Input: part model. Units: mm. Frame: model coordinates. A direction names the side the tool comes from. Round coordinates to 2 decimals unless told otherwise and drop trailing zeros. Loops run counter-clockwise (first coordinate to the right, second up) from the corner with the lowest first, then second, coordinate; pieces in that order, holes last.
1) Draft query along Z for faces 6 (the face through (10.1, -20.7, 5.1)), 7 (the face through (-12.584, -23.813, 5.664)), 8 (the face through (12.584, -23.813, 5.664)), 9 (the face through (12.53, -24.14, 8.1)). Return one class per face: pulls with the +Z half, pulls with the -Z half, needs draft (parallel to the pull), parting line crosses it, or undercut.
2) Access query for faces 1 (the face through (-14.699, 0.843, 0.285)), 2 (the face through (12.53, -19.9, 8.14)), 3 (the face through (14.715, -19.301, 5.014)), 4 (the face through (-10.401, -24.715, 5.014)), 5 (the face through (10.401, -19.285, 4.986)). Directions: +Z, -Z, +X, -X, +Y, -Y. A direction counts if a zero-diameter tool reaches every point of the face in a straight line with its end or side. Return the directions, or none.
3) Section C-C, the plane z = 6.5. State how many separate pieces and enclosed holes the cut face has, and give its area (3 significant figures).
4) First-contact query: pin 1 (3 mm diameter, centred on x = 3.5, y = 6.5, fed in from +Z); pin 2 (1 mm diameter, centred on x = 13, z = 4.5, fed in from +Y); pin 3 (3 mm diameter, centred on x = 4, z = 6, fed in from +Y). Flat tips, straight axial feed; report the tip coordinate or a pass-through.
5) Section B-B, the plane x = 7.5. Return loops of the section in (y, z).
6) Ray query, line 1 along Y through (x, z) = (-12.75, 6); line 2 along Y through (x, z) = (12.5, 4.25); line 3 along Z through (x, y) = (-12.25, 7). Return the intervals inside material, ascending.
from build123d import *

# Parameters (mm, degrees)
SKETCH1_W           = 30
SKETCH1_H           = 50
BOSS_EXTRUDE1_DEPTH = 3
SKETCH2_W           = 4.9
SKETCH2_H           = 6
BOSS_EXTRUDE2_DEPTH = 6
SKETCH3_R           = 1.55
CUT_EXTRUDE1_DEPTH  = 41.074929819
FILLET1_R           = 3
FILLET2_R           = 1


with BuildPart() as part:
    # Sketch1 → Boss-Extrude1 (new body)
    with BuildSketch(Plane.XY):
        Rectangle(SKETCH1_W, SKETCH1_H)
    extrude(amount=BOSS_EXTRUDE1_DEPTH)

    # Sketch2 → Boss-Extrude2 (add)
    with BuildSketch(Plane.XY.offset(3)):
        with Locations((-12.55, -22)):
            Rectangle(SKETCH2_W, SKETCH2_H)
    boss_extrude2 = extrude(amount=BOSS_EXTRUDE2_DEPTH)

    # Sketch3 → Cut-Extrude1 (cut, through all)
    with BuildSketch(Plane.ZY.offset(15)):
        with Locations((6, -22.3)):
            Circle(SKETCH3_R)
    cut_extrude1 = extrude(amount=-CUT_EXTRUDE1_DEPTH, mode=Mode.SUBTRACT)

    # Mirror1: Boss-Extrude2, Cut-Extrude1 across plane
    add(boss_extrude2.mirror(Plane(origin=(0, 0, 0), x_dir=(0, 0, 1), z_dir=(1, 0, 0))))
    add(cut_extrude1.mirror(Plane(origin=(0, 0, 0), x_dir=(0, 0, 1), z_dir=(1, 0, 0))), mode=Mode.SUBTRACT)

    # Fillet1
    fillet1_edges = [part.edges().sort_by_distance(p)[0] for p in [
        (12.55, -19, 9),
        (12.55, -25, 9),
        (-12.55, -19, 9),
        (-12.55, -25, 9),
    ]]
    fillet(fillet1_edges, radius=FILLET1_R - 0.0001)  # a hair under: the kernel refuses the full size

    # Fillet2
    fillet2_edges = [part.edges().sort_by_distance(p)[0] for p in [
        (-15, 3, 3),
        (0, -25, 3),
        (-10.1, -22, 3),
        (-12.55, -19, 3),
        (15, 3, 3),
        (10.1, -22, 3),
        (12.55, -19, 3),
        (0, -25, 0),
        (15, -25, 3.00005),
        (10.1, -25, 4.50005),
        (-10.1, -25, 4.50005),
        (-15, -25, 3.00005),
        (10.1, -19, 4.50005),
        (-15, 0, 0),
        (10.1, -19.878650367, 8.121349633),
        (10.1, -24.121349633, 8.121349633),
        (15, -19, 4.50005),
        (15, -19.878650367, 8.121349633),
        (15, -24.121349633, 8.121349633),
        (-15, -19, 4.50005),
        (-15, -24.121349633, 8.121349633),
        (0, 25, 0),
        (-15, -19.878650367, 8.121349633),
        (-10.1, -19, 4.50005),
        (-10.1, -24.121349633, 8.121349633),
        (-10.1, -19.878650367, 8.121349633),
        (15, 0, 0),
        (0, 25, 3),
    ]]
    fillet(fillet2_edges, radius=FILLET2_R)


solid = part.part
Final values:
1. face 6: needs draft
1. face 7: undercut
1. face 8: undercut
1. face 9: pulls with the +Z half
2. face 1: -Z, -X, +Y, -Y
2. face 2: +Z, +X, -X, +Y
2. face 3: +Z, +X, +Y
2. face 4: +Z, -Y
2. face 5: +Z, +Y
3. separate pieces: 4
3. enclosed holes: 0
3. area: 27.5 mm2
4. pin 1: stops at z = 3
4. pin 2: stops at y = -19
4. pin 3: passes through
5. outline: (-25, 1) arc R1 ccw to (-24, 0) - (24, 0) arc R1 ccw to (25, 1) - (25, 2) arc R1 ccw to (24, 3) - (-24, 3) arc R1 ccw to (-25, 2) - close
6. line 1: y = -25 to -23.85, -20.75 to -19
6. line 2: y = -25 to -19
6. line 3: z = 0 to 3
